Build history of the part. All positions in model axes, mm. A direction names the side the tool comes from. Give positions to 0.01 mm unless a question says otherwise; leave off trailing zeros. Loops run counter-clockwise (first coordinate to the right, second up) from the corner with the lowest first, then second, coordinate; pieces in that order, holes last. Notation, with made-up numbers: (81.5, 89.25) -> (116.5, 89.25) arc R19 cw to (116.5, 100.25) -> close; hole circle Ø10 at (56.5, 48.5). An arc over 180 degrees is marked (long way). Answer as a JSON object with one key per item and string values. Group by question number.
from build123d import *
from OCP.BRepAlgoAPI import BRepAlgoAPI_Cut
from OCP.TopTools import TopTools_ListOfShape

# Parameters (mm, degrees)
SKETCH2_W          = 408.49124402
SKETCH2_H          = 323.52250017
CUT_EXTRUDE1_DEPTH = 68.1736
SKETCH3_W          = 76.2
SKETCH3_H          = 76.2
CUT_EXTRUDE2_DEPTH = 38.1
SKETCH5_W          = 393.276963666
SKETCH5_H          = 361.967680156
CUT_EXTRUDE4_DEPTH = 29.21


with BuildPart() as part:
    # Sketch1 → Revolve1 (revolve)
    with BuildSketch(Plane.XY):
        with BuildLine():
            Line((0, 152.4), (0, -152.4))
            ThreePointArc((0, -152.4), (152.4, 0), (0, 152.4))
        make_face()
    revolve(axis=Axis((0, 152.4, 0), (0, -1, 0)))

    # Sketch2 → Cut-Extrude1 (cut)
    with BuildSketch(Plane(origin=(0, 152.4, 0), x_dir=(1, 0, 0), z_dir=(0, 1, 0))):
        Rectangle(SKETCH2_W, SKETCH2_H)
    extrude(amount=-CUT_EXTRUDE1_DEPTH, mode=Mode.SUBTRACT)


with BuildPart() as cut_extrude2_tool:
    # Sketch3 → Cut-Extrude2 (new body)
    with BuildSketch(Plane(origin=(0, -152.4, 0), x_dir=(-1, 0, 0), z_dir=(0, -1, 0))):
        Rectangle(SKETCH3_W, SKETCH3_H)
    extrude(amount=-CUT_EXTRUDE2_DEPTH)


with BuildPart() as part_1:
    add(part.part)

    # Cut-Extrude2: cut by cut_extrude2_tool, with a tolerance
    cut_extrude2_stock = TopTools_ListOfShape()
    cut_extrude2_stock.Append(part_1.part.wrapped)
    cut_extrude2_tools = TopTools_ListOfShape()
    cut_extrude2_tools.Append(cut_extrude2_tool.part.wrapped)
    cut_extrude2_cut = BRepAlgoAPI_Cut()
    cut_extrude2_cut.SetArguments(cut_extrude2_stock)
    cut_extrude2_cut.SetTools(cut_extrude2_tools)
    cut_extrude2_cut.SetFuzzyValue(0.00001)
    cut_extrude2_cut.Build()
    add(Compound.cast(cut_extrude2_cut.Shape()).solids(), mode=Mode.REPLACE)

    # Sketch5 → Cut-Extrude4 (cut)
    with BuildSketch(Plane(origin=(0, -152.4, 0), x_dir=(-1, 0, 0), z_dir=(0, -1, 0))):
        Rectangle(SKETCH5_W, SKETCH5_H)
    extrude(amount=-CUT_EXTRUDE4_DEPTH, mode=Mode.SUBTRACT)


solid = part_1.part
(1) Saw through at B-B on z = 28. List the corners of the cut face in (x, y).
(2) Saw through at D-D on x = -106. List the corners of the cut face in (y, z).
(3) 3-axis set-ups, long thin cutter, end or side, ignore diameter. For faces 1 (the flat face through (1, -123.19, 39)), 2 (the flat face through (1, -114.3, -1)): which of +Z, -Z, +X, -X, +Y, -Y reach the whole face in a straight line?
(4) Pin check, flat tips, straight feed: pin 1 (4.5 mm diameter, centred on x = 1.5, y = -118.5, fed in from +Z); pin 2 (12 mm diameter, centred on x = -51.5, z = -116.5, fed in from -Y); pin 3 (4.5 mm diameter, centred on y = -118, z = 9, fed in from +X). Stop position of each tip, or through.
(5) Saw through at C-C on y = -96. List the corners of the cut face in (x, z).
(6) Pull direction Z, two halves, no side cores. Call faces 3 (the flat face through (-38.1, -119, 1)), 4 (the flat face through (38.1, -119, 1)), 5 (the flat face through (-2, 84.226, -2)): pulls with the +Z half, pulls with the -Z half, needs draft (parallel to the pull), parting line crosses it, or undercut.
(7) Saw through at A-A on x = 21.5. List the corners of the cut face in (y, z).
(8) Probe line 1 along Y through (x, z) = (54, 99); line 2 along X through (y, z) = (60, -4.5); line 3 along X through (y, z) = (-103.5, 73.5). List the from-to ranges inside material, lowest first. Write a range as [from, to].
Calculated:
{
 "1": {"outline": "(-123.89, 84.23) arc R149.81 ccw to (-85.24, -123.19) -> (-38.1, -123.19) -> (-38.1, -114.3) -> (38.1, -114.3) -> (38.1, -123.19) -> (85.24, -123.19) arc R149.81 ccw to (123.89, 84.23) -> close"},
 "2": {"outline": "(84.23, -69.97) -> (84.23, 69.97) arc R109.5 ccw (long way) to start"},
 "3": {"face 1": "+Z, -Z, +X, -X, -Y", "face 2": "-Y"},
 "4": {"pin 1": "stops at z = 98.54", "pin 2": "stops at y = -92.16", "pin 3": "stops at x = 98.73"},
 "5": {"outline": "circle Ø236.73 at (0, 0)"},
 "6": {"face 3": "undercut", "face 4": "undercut", "face 5": "needs draft"},
 "7": {"outline": "(-123.19, -87.11) arc R150.88 ccw to (84.23, -125.18) -> (84.23, 125.18) arc R150.88 ccw to (-123.19, 87.11) -> (-123.19, 38.1) -> (-114.3, 38.1) -> (-114.3, -38.1) -> (-123.19, -38.1) -> close"},
 "8": {"line 1": "y = [-102.51, 84.23]", "line 2": "x = [-140.02, 140.02]", "line 3": "x = [-84.33, 84.33]"}
}
